```python
from build123d import *

# Parameters (mm, degrees)
SKETCH1_R               = 3
BOSS_EXTRUDE1_DEPTH     = 50
CUT_EXTRUDE1_DEPTH      = 236.677746086
CUT_EXTRUDE1_DEPTH_BACK = 236.677746086
SKETCH2_W               = 220
SKETCH2_H               = 40
SKETCH3_W               = 10
SKETCH3_H               = 5
BOSS_EXTRUDE2_DEPTH     = 10
CUT_EXTRUDE2_REACH      = 237.678
SKETCH4_W               = 7
SKETCH4_H               = 5
FILLET1_R               = 2
SKETCH5_R               = 1.5
CUT_EXTRUDE3_DEPTH      = 10


with BuildPart() as part:
    # Sketch1 → Boss-Extrude1 (new body)
    with BuildSketch(Plane.XY):
        with BuildLine():
            Line((124.16515139, 0), (230, 0))
            Line((230, 0), (230, 5))
            Line((230, 5), (124.16515139, 5))
            ThreePointArc((124.16515139, 5), (115, 12), (105.83484861, 5))
            Line((105.83484861, 5), (0, 5))
            Line((0, 5), (0, 0))
            Line((0, 0), (105.83484861, 0))
            ThreePointArc((105.83484861, 0), (115, -7), (124.16515139, 0))
        make_face()
        with Locations((115, 2.5)):
            Circle(SKETCH1_R, mode=Mode.SUBTRACT)
    extrude(amount=BOSS_EXTRUDE1_DEPTH)

    # Sketch2 → Cut-Extrude1 (cut, two sides: drawn at the far end of the back side and taken through both)
    with BuildSketch(Plane(origin=(0, 0, 0), x_dir=(-1, 0, 0), z_dir=(0, -1, 0)).offset(-CUT_EXTRUDE1_DEPTH_BACK)):
        with Locations((-115, -25)):
            Rectangle(SKETCH2_W, SKETCH2_H)
    extrude(amount=CUT_EXTRUDE1_DEPTH + CUT_EXTRUDE1_DEPTH_BACK, mode=Mode.SUBTRACT)

    # Sketch3 → Boss-Extrude2 (add)
    with BuildSketch(Plane(origin=(5, 0, 0), x_dir=(0, 0, -1), z_dir=(1, 0, 0))):
        with Locations((-25, 2.5)):
            Rectangle(SKETCH3_W, SKETCH3_H)
    extrude(amount=BOSS_EXTRUDE2_DEPTH)

    # Sketch4 → Cut-Extrude2 (cut, up to next)
    with BuildSketch(Plane(origin=(0, 5, 0), x_dir=(1, 0, 0), z_dir=(0, 1, 0)), mode=Mode.PRIVATE) as cut_extrude2_sk1:
        with Locations((11.5, -25)):
            Rectangle(SKETCH4_W, SKETCH4_H)
    cut_extrude2_tool1 = extrude(cut_extrude2_sk1.sketch, amount=-CUT_EXTRUDE2_REACH, mode=Mode.PRIVATE) & part.part
    add(cut_extrude2_tool1.solids().sort_by_distance((11.5, 5, 25))[0], mode=Mode.SUBTRACT)

    # Fillet1
    fillet1_edges = [part.edges().sort_by_distance(p)[0] for p in [
        (5, 2.5, 30),
        (5, 2.5, 20),
    ]]
    fillet(fillet1_edges, radius=FILLET1_R)

    # Sketch5 → Cut-Extrude3 (cut)
    with BuildSketch(Plane(origin=(0, 0, 20), x_dir=(-1, 0, 0), z_dir=(0, 0, -1))):
        with Locations((-12, 2.5)):
            Circle(SKETCH5_R)
    extrude(amount=-CUT_EXTRUDE3_DEPTH, mode=Mode.SUBTRACT)


solid = part.part
```
Geometry: final body of the model. Coordinates: model frame, mm. A direction names the side the tool comes from. Round coordinates to 2 decimals unless told otherwise and drop trailing zeros. Order: outer loops, then holes, each group sorted by start corner. A loop starts at its lowest first (then second) coordinate and runs counter-clockwise, first axis right, second up. Notation, with made-up numbers: M 76,66.5 L 108,66.5 A18 cw 108,79.5 Z; hole C 76,36.5 d8. An arc over 180 degrees is marked long. Use one line per item in the form item = value. Start each with the question number.
Q1. Cut plane B-B (x = 164). Return loops of the section in (y, z).
Q2. Access query for faces 4 (the face through (185.2, 5, 45.3)), 5 (the face through (5, 3, 12)), 6 (the face through (45.3, 5, 45.3)). Directions: +Z, -Z, +X, -X, +Y, -Y. A direction counts if a zero-diameter tool reaches every point of the face in a straight line with its end or side. Return the directions, or none.
Q3. Cut plane A-A (z = 25). Return loops of the section in (x, y), and give its area (3 significant figures).
Q4. Mould query, pull axis Z, two halves, no side actions, for faces 1 (the face through (10, 2, 30)), 2 (the face through (113, -2, 0)), 3 (the face through (184.7, 0, 45.3)). Classes: +Z half, -Z half, draft (parallel to the pull), parting line (faces both ways), or undercut.
Q5. Material intervals for line 1 (X direction, y = 3.5, z = 14); line 2 (X direction, y = 3, z = 29); line 3 (Y direction, x = 115, z = 48), sorted ascending. Write a range as [from, to].
Q6. Pin query (flat end, axial travel): pin 1 Ø5.5 at (x, y) = (115, 2.5) entering from +Z. Return the tip coordinate at first contact, or that it passes through.
Geometry results:
q1.outline = M 0,0 L 5,0 L 5,5 L 0,5 Z; M 0,45 L 5,45 L 5,50 L 0,50 Z
q2.face_4 = +Z, -Z, +X, +Y
q2.face_5 = +Y, -Y
q2.face_6 = +Z, -Z, -X, +Y
q3.outline = M 0,0 L 8,0 L 8,5 L 0,5 Z; M 225,0 L 230,0 L 230,5 L 225,5 Z
q3.area = 65.0 mm^2
q4.face_1 = undercut
q4.face_2 = -Z half
q4.face_3 = draft
q5.line_1 = [0, 5], [225, 230]
q5.line_2 = [0, 10.59], [13.41, 15], [225, 230]
q5.line_3 = [-7, -0.5], [5.5, 12]
q6.pin_1 = through
